Verification items for this drawing (mm, ordinates from the low corner). Coordinates: 2 decimals unless noted, no trailing zeros. Order: outer loops, then holes, each group sorted by start corner. A loop starts at its lowest first (then second) coordinate and runs counter-clockwise, first axis right, second up. Notation, with made-up numbers: M 3,13 L 9,13 A22 cw 9,36 Z; hole C 62,3.5 d2. An arc over 180 degrees is marked long. Answer as a JSON object with one key per item and string values. Group by question number.
(1) Cross-section at B-B (y = 756). Enter the section's corners in (x, z).
(2) Gauge pin test, flat end, axial feed: pin 1 Ø1.5 at (y, z) = (729.5, 20.5) entering from -X. Record the tip position at first contact, or that the pin passes through.
(3) Cross-section at A-A (z = 9.5). Enter the section's corners in (x, y) (3 decimals), plus the area to 3 significant figures.
(4) Material ranges on line 1 (X direction, y = 768, z = 14.5); line 2 (X direction, y = 161.5, z = 9), recorded low to high.
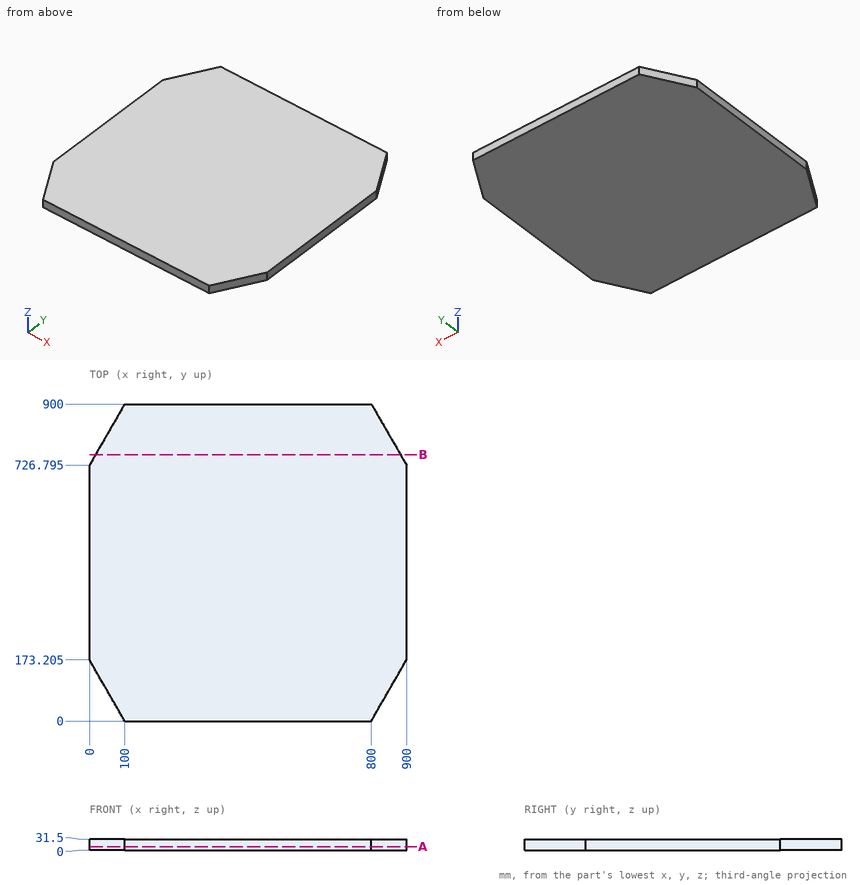
Taken from the geometry:
{
 "1": {"outline": "M 16.86,0 L 883.14,0 L 883.14,31.5 L 16.86,31.5 Z"},
 "2": {"pin 1": "stops at x = 1.13"},
 "3": {"outline": "M 0,173.205 L 100,0 L 800,0 L 900,173.205 L 900,726.795 L 800,900 L 100,900 L 0,726.795 Z", "area": "775,000 mm²"},
 "4": {"line 1": "x = 23.79 to 876.21", "line 2": "x = 6.76 to 893.24"}
}
